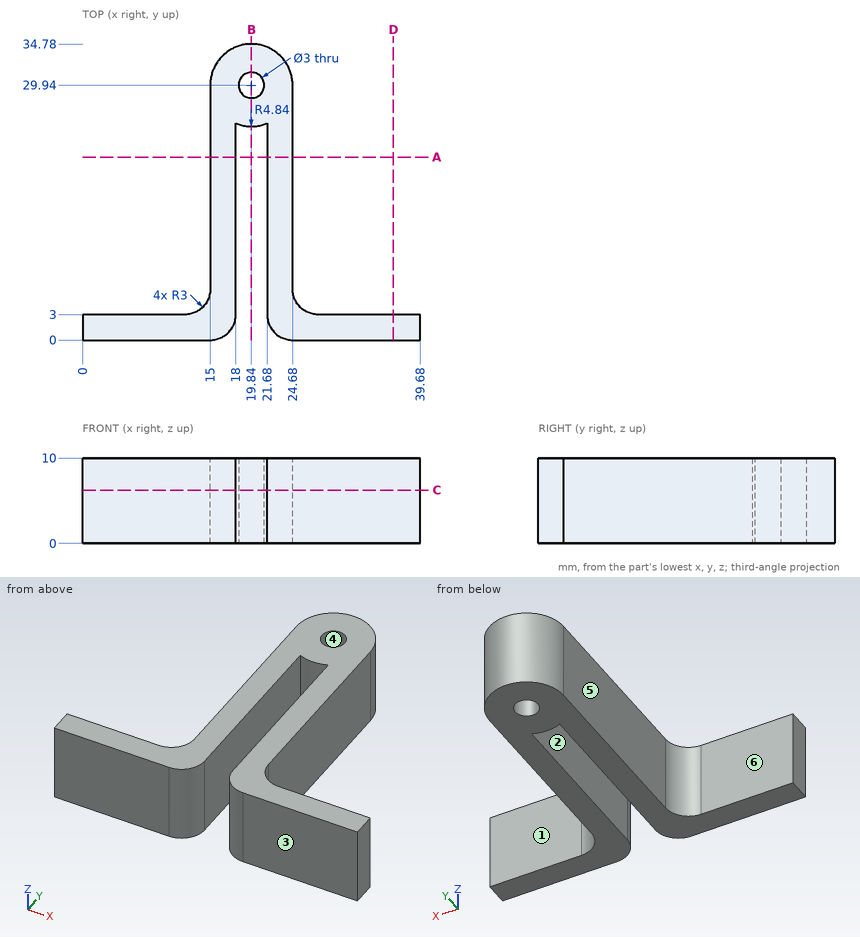
Can you work these out from the drawing? Everything is in mm from the part's minimum corner. A direction names the side the tool comes from. Give positions to 0.01 mm unless a question says otherwise; leave off trailing zeros. Loops run counter-clockwise (first coordinate to the right, second up) from the corner with the lowest first, then second, coordinate; pieces in that order, holes last. Notation, with made-up numbers: (89.5, -23) -> (104.5, -23) arc R27 ccw to (104.5, 9) -> close; hole circle Ø10 at (77.25, 22.5). An arc over 180 degrees is marked (long way). Return JSON: item names as keys, results as strings.
Item 1: If we section it at A-A on y = 21.5: List the corners of the cut face in (x, z) for me.
Geometry results:
{"outline": "(15, 0) -> (18, 0) -> (18, 10) -> (15, 10) -> close; (21.68, 0) -> (24.68, 0) -> (24.68, 10) -> (21.68, 10) -> close"}
Item 2: I need wall thicknesses on L1, parallel to X at y = 22.5, z = 4; L2, parallel to Y at x = 19.84, z = 4; L3, parallel to X at y = 30, z = 2. Which ranges of each line are inside material? Lowest first, please. Write a range as from..to.
Geometry results:
{"L1": "x = 15..18, 21.68..24.68", "L2": "y = 25.1..28.44, 31.44..34.78", "L3": "x = 15..18.34, 21.34..24.68"}
Item 3: Which directions (+Z, -Z, +X, -X, +Y, -Y) give clear straight access to the entire face, cutting with the end or side of a thin tool? Please do the marked faces 1, 2 and 3.
Geometry results:
{"face 1": "+Z, -Z, +X, +Y", "face 2": "+Z, -Z, -Y", "face 3": "+Z, -Z, +X, -X, -Y"}
Item 4: If we section it at C-C on z = 6.25: List the corners of the cut face in (x, y) for me.
Geometry results:
{"outline": "(0, 0) -> (15, 0) arc R3 ccw to (18, 3) -> (18, 25.46) arc R4.84 ccw to (21.68, 25.46) -> (21.68, 3) arc R3 ccw to (24.68, 0) -> (39.68, 0) -> (39.68, 3) -> (27.68, 3) arc R3 cw to (24.68, 6) -> (24.68, 29.94) arc R4.84 ccw to (15, 29.94) -> (15, 6) arc R3 cw to (12, 3) -> (0, 3) -> close; hole circle Ø3 at (19.84, 29.94)"}
Item 5: I'm going to push flat-ended pins straight in: pin 1 (5 mm diameter, centred on y = 30, z = 8, fed in from +X); pin 2 (4 mm diameter, centred on x = 26.5, z = 5.5, fed in from -Y); pin 3 (3 mm diameter, centred on x = 5.5, z = 7.5, fed in from +Y); pin 4 (5 mm diameter, centred on y = 18.5, z = 5.5, fed in from -X). Where does each tip first touch, or does it pass through?
Geometry results:
{"pin 1": "stops at x = 24.68", "pin 2": "stops at y = 0", "pin 3": "stops at y = 3", "pin 4": "stops at x = 15"}
Item 6: If we section it at D-D on x = 36.5: List the corners of the cut face in (y, z) for me.
Geometry results:
{"outline": "(0, 0) -> (3, 0) -> (3, 10) -> (0, 10) -> close"}
Item 7: We'd pull the mould along Y, two halves only. Please class the marked faces 4, 5 and 6: +Y half, -Y half, draft (parallel to the pull), parting line (faces both ways), or undercut.
Geometry results:
{"face 4": "undercut", "face 5": "draft", "face 6": "+Y half"}
Item 8: If we section it at B-B on x = 19.84: List the corners of the cut face in (y, z) for me.
Geometry results:
{"outline": "(25.1, 0) -> (28.44, 0) -> (28.44, 10) -> (25.1, 10) -> close; (31.44, 0) -> (34.78, 0) -> (34.78, 10) -> (31.44, 10) -> close"}
